For this review, take the finished solid that the model builds, in its own axes (mm). Round coordinates to 2 decimals unless told otherwise and drop trailing zeros. Loops run counter-clockwise (first coordinate to the right, second up) from the corner with the lowest first, then second, coordinate; pieces in that order, holes last. Notation, with made-up numbers: M 32,16 L 38,16 A28 ccw 38,45 Z; hole C 3,-1 d1. An arc over 180 degrees is marked long. Write item = value, one per line. Start each with the question number.
Autodesk Inventor part; units mm, degrees
ref_plane "YZ Plane" through (0, 0, 0) normal (1, 0, 0) x (0, 1, 0)
ref_plane "XZ Plane" through (0, 0, 0) normal (0, 1, 0) x (-1, 0, 0)
ref_plane "XY Plane" through (0, 0, 0) normal (0, 0, 1) x (1, 0, 0)
ref_plane "Work Plane1" through (189.9024, 510.8101, -163.2862) normal (-1, 0, 0) x (0, 0, 1)
sketch "Sketch1" plane through (189.9024, 510.8101, -163.2862) normal (-1, 0, 0) x (0, 0, 1)
  arc A0 (-25.9275, -325.719) -> (-33.9275, -333.719) centre (-25.9275, -333.719) ccw
  line L0 (-25.9275, -325.719) -> (1.0727, -325.719)
  arc A1 (1.0727, -325.719) -> (3.0415, -325.473) centre (1.0727, -317.719) ccw
  line L1 (3.0415, -325.473) -> (116.1034, -296.7651)
  arc A2 (118.0722, -296.519) -> (116.1034, -296.7651) centre (118.0722, -304.519) ccw
  line L2 (118.0722, -296.519) -> (174.0725, -296.519)
  arc A3 (182.0725, -304.519) -> (174.0725, -296.519) centre (174.0725, -304.519) ccw
  line L3 (182.0725, -304.519) -> (182.0725, -380.5983)
  arc A4 (176.4102, -388.2491) -> (182.0725, -380.5983) centre (174.0725, -380.5983) ccw
  line L4 (176.4102, -388.2491) -> (3.2153, -441.1698)
  arc A5 (0.8775, -441.519) -> (3.2153, -441.1698) centre (0.8775, -433.519) ccw
  line L5 (-33.9275, -403.519) -> (-33.9275, -333.719)
  circle A6 centre (104.0232, -361.3682) radius 2.25
  circle A7 centre (133.7217, -331.6698) radius 2.25
  circle A8 centre (166.0725, -329.019) radius 2.75
  circle A9 centre (118.8725, -346.519) radius 12
  circle A10 centre (142.4425, -322.949) radius 2.5
  circle A11 centre (-26.9275, -434.819) radius 2.25
  circle A12 centre (-26.9275, -358.419) radius 2.25
  circle A13 centre (-0.9275, -332.419) radius 2.25
  circle A14 centre (-0.9275, -358.419) radius 2.25
  circle A15 centre (71.6725, -346.519) radius 6.05
  circle A16 centre (166.0725, -346.519) radius 6.05
  circle A17 centre (-26.9275, -332.419) radius 2.25
  circle A18 centre (-26.9275, -408.819) radius 2.25
  circle A19 centre (142.4425, -370.089) radius 2.5
  circle A20 centre (95.3025, -370.089) radius 2.5
  circle A21 centre (166.0725, -364.019) radius 2.75
  circle A22 centre (71.6725, -364.019) radius 2.75
  circle A23 centre (133.7217, -361.3682) radius 2.25
  circle A24 centre (104.0232, -331.6698) radius 2.25
  circle A25 centre (71.6725, -329.019) radius 2.75
  circle A26 centre (95.3025, -322.949) radius 2.5
  arc A27 (-81.9275, -405.519) -> (-83.9275, -407.519) centre (-81.9275, -407.519) ccw
  line L6 (-81.9275, -405.519) -> (-35.9275, -405.519)
  arc A28 (-35.9275, -405.519) -> (-33.9275, -403.519) centre (-35.9275, -403.519) ccw
  line L7 (0.8775, -441.519) -> (-81.9275, -441.519)
  arc A29 (-83.9275, -439.519) -> (-81.9275, -441.519) centre (-81.9275, -439.519) ccw
  line L8 (-83.9275, -439.519) -> (-83.9275, -407.519)
  circle A30 centre (-76.4275, -411.519) radius 2.75
  circle A31 centre (-76.4275, -435.519) radius 2.75
  circle A32 centre (-0.9275, -408.819) radius 2.25
  circle A33 centre (-0.9275, -434.819) radius 2.25
  circle A34 centre (-41.4275, -435.519) radius 2.75
  circle A35 centre (-41.4275, -411.519) radius 2.75
  point P0 (163.2862, -510.8101)
  point P1 (-25.9275, -122.4465)
sketch "Sketch2" plane through (189.9024, 510.8101, -163.2862) normal (-1, 0, 0) x (0, 0, 1)
  line L0 (176.4102, -388.2491) -> (3.2153, -441.1698)
  arc A0 (-25.9275, -325.719) -> (-33.9275, -333.719) centre (-25.9275, -333.719) ccw
  line L1 (-25.9275, -325.719) -> (1.0727, -325.719)
  arc A1 (1.0727, -325.719) -> (3.0415, -325.473) centre (1.0727, -317.719) ccw
  line L2 (3.0415, -325.473) -> (116.1034, -296.7651)
  circle A2 centre (-0.9275, -332.419) radius 2.25
  circle A3 centre (-0.9275, -358.419) radius 2.25
  circle A4 centre (-26.9275, -332.419) radius 2.25
  circle A5 centre (-26.9275, -358.419) radius 2.25
  arc A6 (0.8775, -441.519) -> (3.2153, -441.1698) centre (0.8775, -433.519) ccw
  circle A7 centre (-26.9275, -434.819) radius 2.25
  circle A8 centre (-26.9275, -408.819) radius 2.25
  line L3 (118.0722, -296.519) -> (174.0725, -296.519)
  arc A9 (182.0725, -304.519) -> (174.0725, -296.519) centre (174.0725, -304.519) ccw
  line L4 (182.0725, -304.519) -> (182.0725, -380.5983)
  arc A10 (176.4102, -388.2491) -> (182.0725, -380.5983) centre (174.0725, -380.5983) ccw
  arc A11 (118.0722, -296.519) -> (116.1034, -296.7651) centre (118.0722, -304.519) ccw
  circle A12 centre (166.0725, -346.519) radius 6.05
  circle A13 centre (166.0725, -364.019) radius 2.75
  circle A14 centre (166.0725, -329.019) radius 2.75
  circle A15 centre (71.6725, -329.019) radius 2.75
  circle A16 centre (71.6725, -364.019) radius 2.75
  circle A17 centre (71.6725, -346.519) radius 6.05
  circle A18 centre (118.8725, -346.519) radius 17.5 construction
  circle A19 centre (131.2468, -334.1446) radius 1.75
  circle A20 centre (106.4981, -334.1446) radius 1.75
  circle A21 centre (106.4981, -358.8934) radius 1.75
  circle A22 centre (131.2468, -358.8934) radius 1.75
  circle A23 centre (118.8725, -346.519) radius 6
  arc A24 (-35.9275, -405.519) -> (-33.9275, -403.519) centre (-35.9275, -403.519) ccw
  line L5 (-33.9275, -403.519) -> (-33.9275, -333.719)
  circle A25 centre (-41.4275, -411.519) radius 2.75
  circle A26 centre (-41.4275, -435.519) radius 2.75
  line L6 (-81.9275, -405.519) -> (-35.9275, -405.519)
  line L7 (0.8775, -441.519) -> (-81.9275, -441.519)
  circle A27 centre (-76.4275, -411.519) radius 2.75
  arc A28 (-81.9275, -405.519) -> (-83.9275, -407.519) centre (-81.9275, -407.519) ccw
  circle A29 centre (-76.4275, -435.519) radius 2.75
  line L8 (-83.9275, -439.519) -> (-83.9275, -407.519)
  arc A30 (-83.9275, -439.519) -> (-81.9275, -441.519) centre (-81.9275, -439.519) ccw
  circle A31 centre (-0.9275, -88.6017) radius 2.15
  circle A32 centre (-0.9275, -114.6017) radius 2.15
  circle A33 centre (-0.9275, -408.819) radius 2.25
  circle A34 centre (-0.9275, -434.819) radius 2.25
  point P0 (163.2862, -510.8101)
  point P1 (-25.9275, -122.4465)
  point P2 (163.2862, -510.8101)
  point P3 (-0.9275, -434.819)
  dimension "d2" = 35
  dimension "d3" = 3.5
  dimension "d4" = 90
  dimension "d5" = 12
extrude "Extrusion2" add sketch "Sketch2" along normal blind 6 contours L0 A6 L7 A30 L8 A28 L6 A24 L5 A0 L1 A1 L2 A11 L3 A9 L4 A10
properties part number "SIDE_SUPPORT_PLATE-PASSIVE"
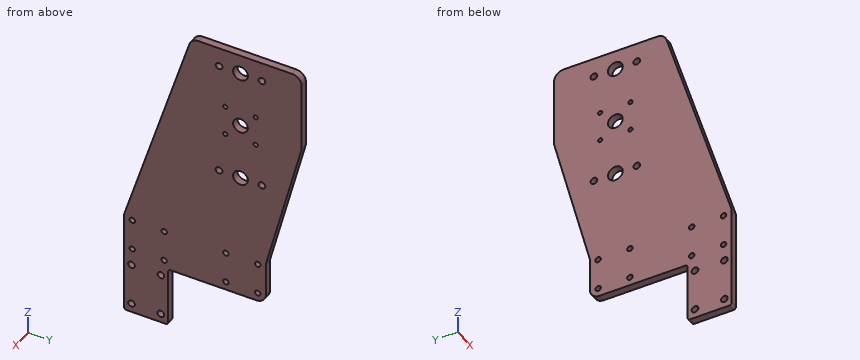
(1) For pin 1 Ø1.8 at (x, y) = (187, 157.5) entering from -Z; pin 2 Ø5 at (y, z) = (152.39, -190.21) entering from +X; pin 3 Ø1.8 at (x, z) = (186.5, -182) entering from +Y, all flat-tipped, find the tip position at first contact; note any pin that passes through.
(2) Add section A-A on y = 191. Write out the cut boundary in (x, z).
(3) Wall thickness on L1, parallel to Z at x = 184.9, y = 160; L2, parallel to Z at x = 184.8, y = 176; L3, parallel to Z at x = 185.25, y = 145.5: over which ranges is each line inside the solid? List them lowest first.
(4) Add section C-C on z = -117. Write out the cut boundary in (x, y).
(5) Add section B-B on x = 186.45. Count the separate pieces of the cut face and the enclosed holes in it, and give its area (3 significant figures).
Answer sheet:
q1.pin_1 = -197.21
q1.pin_2 = 189.9
q1.pin_3 = 185.09
q2.outline = M 183.9,-137.94 L 189.9,-137.94 L 189.9,18.79 L 183.9,18.79 Z
q3.L1 = -197.21 to -95.88, -87.35 to -48.61, -40.22 to -1.48, 7.05 to 18.79
q3.L2 = -197.21 to -58.41, -55.17 to -33.66, -30.42 to 18.79
q3.L3 = -197.21 to -94.04, -89.19 to 0.36, 5.21 to 18.79
q4.outline = M 183.9,82.8 L 189.9,82.8 L 189.9,196.32 L 183.9,196.32 Z
q5.separate_pieces = 1
q5.enclosed_holes = 23
q5.area = 24,700 mm²
